```python
from build123d import *

# Parameters (mm, degrees)
SKETCH2_W                    = 120.65
SKETCH2_H                    = 1.5875
BASE_FLANGE1_DEPTH           = 25.4
EDGE_FLANGE1_STRIP_W         = 16.51
EDGE_FLANGE1_STRIP_H         = 1.5875
EDGE_FLANGE1_STRIP_CUT_DEPTH = 120.65
EDGE_FLANGE1_DEPTH           = 120.65
FILLET1_R                    = 2.54
CUT_EXTRUDE1_DEPTH           = 138.966445762
SKETCH11_R                   = 2.15265
CUT_EXTRUDE2_DEPTH           = 139.404146095


# Sheet-metal steps are written as plain solids
with BuildPart() as part:
    # Sketch2 → Base-Flange1 (new body)
    with BuildSketch(Plane(origin=(0, 0, 0), x_dir=(1, 0, 0), z_dir=(0, 1, 0))):
        with Locations((60.325, -0.79375)):
            Rectangle(SKETCH2_W, SKETCH2_H)
    extrude(amount=BASE_FLANGE1_DEPTH)

    # Edge-Flange1 strip (across the edge) → Edge-Flange1 strip cut (cut)
    with BuildSketch(Plane(origin=(120.65, 25.4, 1.5875), x_dir=(0, -1, 0), z_dir=(-1, 0, 0))):
        with Locations((-1.5875, -0.79375)):
            Rectangle(EDGE_FLANGE1_STRIP_W, EDGE_FLANGE1_STRIP_H)
    extrude(amount=EDGE_FLANGE1_STRIP_CUT_DEPTH, mode=Mode.SUBTRACT)

    # Edge-Flange1 section (across the edge) → Edge-Flange1 (add)
    with BuildSketch(Plane(origin=(120.65, 25.4, 1.5875), x_dir=(0, -1, 0), z_dir=(-1, 0, 0))):
        with BuildLine():
            Line((0, 5.08), (0, 61.9125))
            Line((0, 61.9125), (1.5875, 61.9125))
            Line((1.5875, 61.9125), (1.5875, 5.08))
            ThreePointArc((1.5875, 5.08), (3.075397552, 1.487897552), (6.6675, 0))
            Line((6.6675, 0), (6.6675, -1.5875))
            ThreePointArc((6.6675, -1.5875), (1.952865536, 0.365365536), (0, 5.08))
        make_face()
    extrude(amount=EDGE_FLANGE1_DEPTH)

    # Fillet1
    fillet1_edges = [part.edges().sort_by_distance(p)[0] for p in [
        (120.65, 24.60625, 63.5),
        (0, 24.60625, 63.5),
        (0, 0, 0.79375),
        (120.65, 0, 0.79375),
    ]]
    fillet(fillet1_edges, radius=FILLET1_R)

    # Sketch10 → Cut-Extrude1 (cut, through all)
    with BuildSketch(Plane.XY.offset(1.5875)):
        with BuildLine():
            Line((7.112, 8.50265), (8.382, 8.50265))
            ThreePointArc((8.382, 8.50265), (10.53465, 6.35), (8.382, 4.19735))
            Line((8.382, 4.19735), (7.112, 4.19735))
            ThreePointArc((7.112, 4.19735), (4.95935, 6.35), (7.112, 8.50265))
        make_face()
        with BuildLine():
            Line((112.268, 8.50265), (113.538, 8.50265))
            ThreePointArc((113.538, 8.50265), (115.69065, 6.35), (113.538, 4.19735))
            Line((113.538, 4.19735), (112.268, 4.19735))
            ThreePointArc((112.268, 4.19735), (110.11535, 6.35), (112.268, 8.50265))
        make_face()
    extrude(amount=-CUT_EXTRUDE1_DEPTH, mode=Mode.SUBTRACT)

    # Sketch11 → Cut-Extrude2 (cut, through all)
    with BuildSketch(Plane.XZ.offset(-23.8125)):
        with Locations(Location((22.225, 50.8, 0), (0, 0, 270))):
            Circle(SKETCH11_R)
        with Locations(Location((98.425, 50.8, 0), (0, 0, 270))):
            Circle(SKETCH11_R)
    extrude(amount=-CUT_EXTRUDE2_DEPTH, mode=Mode.SUBTRACT)


solid = part.part
```
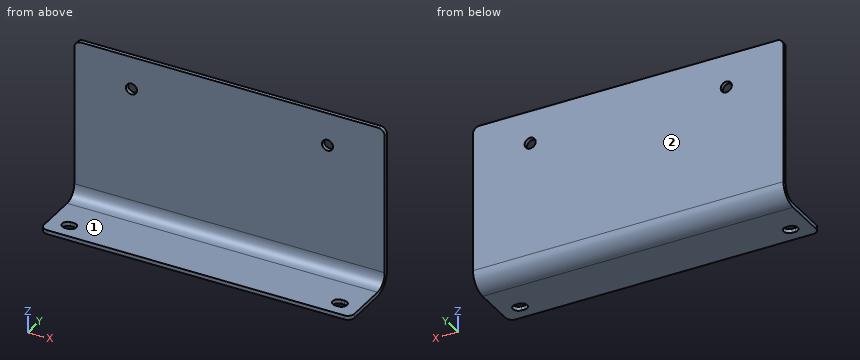
Input: part model. Units: mm. Frame: model coordinates. Face numbers are marked on the shaded views. A direction names the side the tool comes from. Give positions to 0.01 mm unless a question says otherwise; leave off trailing zeros. Order: outer loops, then holes, each group sorted by start corner. A loop starts at its lowest first (then second) coordinate and runs counter-clockwise, first axis right, second up.
1. Section A-A on z = 50.8. Return the cut outline in (x, y).
Derived:
outline: (0, 23.81) - (20.07, 23.81) - (20.07, 25.4) - (0, 25.4) - close; (24.38, 23.81) - (96.27, 23.81) - (96.27, 25.4) - (24.38, 25.4) - close; (100.58, 23.81) - (120.65, 23.81) - (120.65, 25.4) - (100.58, 25.4) - close
2. Section C-C on x = 73. Return the cut outline in (y, z) (1 decimal).
Derived:
outline: (0, 0) - (18.7, 0) arc R6.7 ccw to (25.4, 6.7) - (25.4, 63.5) - (23.8, 63.5) - (23.8, 6.7) arc R5.1 cw to (18.7, 1.6) - (0, 1.6) - close
3. Material intervals for L1, parallel to X at y = 25, z = 50.8; L2, parallel to Z at x = 16.5, y = 10; L3, parallel to Y at x = 33, z = 29, sorted ascending.
Derived:
L1: x = 0 to 20.07, 24.38 to 96.27, 100.58 to 120.65
L2: z = 0 to 1.59
L3: y = 23.81 to 25.4
4. Section B-B on y = 6.35. Return the cut outline in (x, z), and give its area (3 significant figures).
Derived:
outline: (0, 0) - (4.96, 0) - (4.96, 1.59) - (0, 1.59) - close; (10.53, 0) - (110.12, 0) - (110.12, 1.59) - (10.53, 1.59) - close; (115.69, 0) - (120.65, 0) - (120.65, 1.59) - (115.69, 1.59) - close
area: 174 mm2
5. Reachability of the marked faces 1 and 2 from +Z, -Z, +X, -X, +Y, -Y: full face, straight path, thin tool, end or side. Return the list, or none.
Derived:
face 1: +Z, +X, -X, -Y
face 2: +Z, -Z, +X, -X, +Y
6. Section D-D on y = 20.5. Return the cut outline in (x, z).
Derived:
outline: (0, 0.24) - (120.65, 0.24) - (120.65, 1.9) - (0, 1.9) - close
7. Pin query (flat end, axial travel): pin 1 (10 mm diameter, centred on y = 15.5, z = 29, fed in from -X); pin 2 (2 mm diameter, centred on x = 108, z = 53.5, fed in from -Y); pin 3 (1.4 mm diameter, centred on x = 7.5, z = 1, fed in from +Y); pin 4 (1 mm diameter, centred on x = 113, z = 1, fed in from +Y). Return the tip coordinate at first contact, or that it passes through.
Derived:
pin 1: passes through
pin 2: stops at y = 23.81
pin 3: stops at y = 23.18
pin 4: stops at y = 22.95
